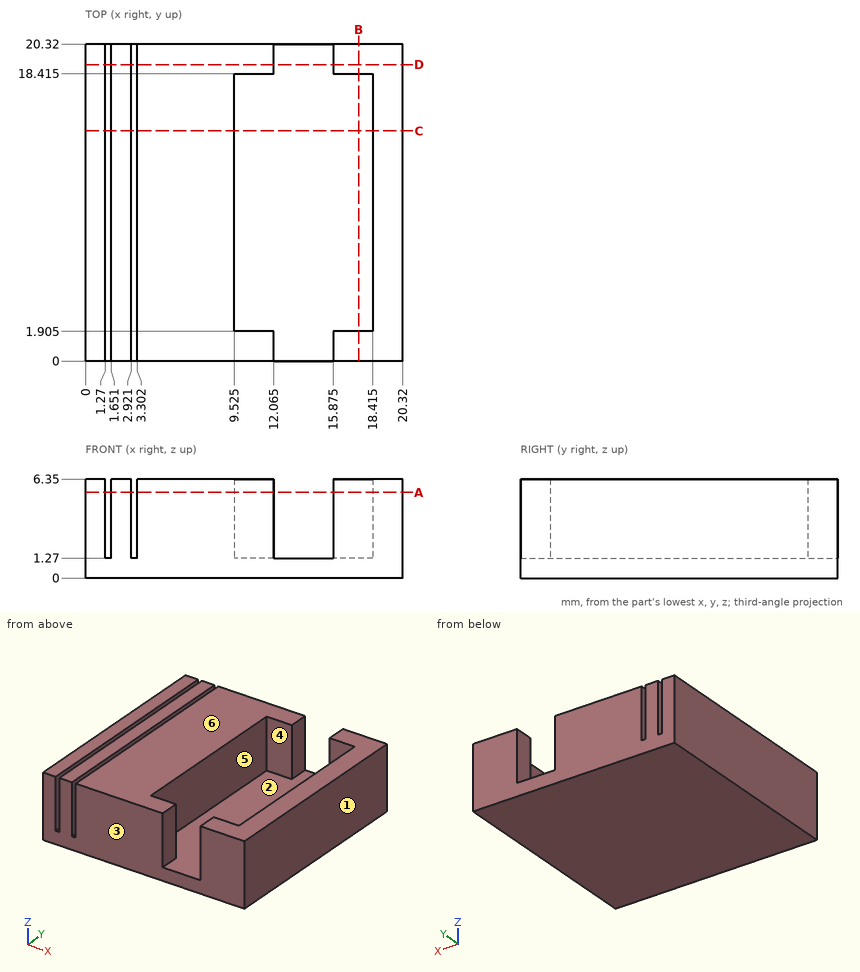
Check sheet for the drawn part. Datum: minimum x, y, z corner. Units: mm. A direction names the side the tool comes from. Give positions to 0.01 mm unless a question says otherwise; leave off trailing zeros. Order: outer loops, then holes, each group sorted by start corner. A loop starts at its lowest first (then second) coordinate and runs counter-clockwise, first axis right, second up. Notation, with made-up numbers: (66.5, -36) -> (83.5, -36) arc R17 ccw to (83.5, -18) -> close; hole circle Ø1 at (-38, -33). An arc over 180 degrees is marked (long way). Return JSON: item names as keys, results as strings.
1. Material ranges on probe 1 along X at (y, z) = (4.25, 5.5) (3 decimals); probe 2 along X at (y, z) = (19.75, 5.75) (3 decimals); probe 3 along Y at (x, z) = (10.5, 2) (3 decimals), recorded low to high. Write a range as [from, to].
From the geometry:
{"probe 1": "[0, 1.27], [1.651, 2.921], [3.302, 9.525], [18.415, 20.32]", "probe 2": "[0, 1.27], [1.651, 2.921], [3.302, 12.065], [15.875, 20.32]", "probe 3": "[0, 1.905], [18.415, 20.32]"}
2. Cross-section at D-D, the plane y = 19. Record the cut outline in (x, z) (3 decimals).
From the geometry:
{"outline": "(0, 0) -> (20.32, 0) -> (20.32, 6.35) -> (15.875, 6.35) -> (15.875, 1.27) -> (12.065, 1.27) -> (12.065, 6.35) -> (3.302, 6.35) -> (3.302, 1.27) -> (2.921, 1.27) -> (2.921, 6.35) -> (1.651, 6.35) -> (1.651, 1.27) -> (1.27, 1.27) -> (1.27, 6.35) -> (0, 6.35) -> close"}
3. Cross-section at A-A, the plane z = 5.5. Record the cut outline in (x, y) (3 decimals).
From the geometry:
{"outline": "(0, 0) -> (1.27, 0) -> (1.27, 20.32) -> (0, 20.32) -> close; (1.651, 0) -> (2.921, 0) -> (2.921, 20.32) -> (1.651, 20.32) -> close; (3.302, 0) -> (12.065, 0) -> (12.065, 1.905) -> (9.525, 1.905) -> (9.525, 18.415) -> (12.065, 18.415) -> (12.065, 20.32) -> (3.302, 20.32) -> close; (15.875, 0) -> (20.32, 0) -> (20.32, 20.32) -> (15.875, 20.32) -> (15.875, 18.415) -> (18.415, 18.415) -> (18.415, 1.905) -> (15.875, 1.905) -> close"}
4. Cross-section at B-B, the plane x = 17.5. Record the cut outline in (y, z) (3 decimals).
From the geometry:
{"outline": "(0, 0) -> (20.32, 0) -> (20.32, 6.35) -> (18.415, 6.35) -> (18.415, 1.27) -> (1.905, 1.27) -> (1.905, 6.35) -> (0, 6.35) -> close"}
5. Set-up check for the marked faces 5 and 6: record each of +Z, -Z, +X, -X, +Y, -Y from which the full face is reachable in a straight line by a thin tool's end or side.
From the geometry:
{"face 5": "+Z", "face 6": "+Z, +X, -X, +Y, -Y"}
6. Mould release check, pull along Y, two halves, no side actions. Record for the marked faces 1, 2, 3 and 4: +Y half, -Y half, draft (parallel to the pull), parting line (faces both ways), or undercut.
From the geometry:
{"face 1": "draft", "face 2": "undercut", "face 3": "-Y half", "face 4": "undercut"}
7. Go/stop test with a flat-tipped pin: P1, Ø5, axis at x = 14.5, y = 12, coming from the +Z side. Record where the tip stops, or that it passes through.
From the geometry:
{"P1": "z = 1.27"}
8. Cross-section at C-C, the plane y = 14.75. Record the cut outline in (x, z) (3 decimals).
From the geometry:
{"outline": "(0, 0) -> (20.32, 0) -> (20.32, 6.35) -> (18.415, 6.35) -> (18.415, 1.27) -> (9.525, 1.27) -> (9.525, 6.35) -> (3.302, 6.35) -> (3.302, 1.27) -> (2.921, 1.27) -> (2.921, 6.35) -> (1.651, 6.35) -> (1.651, 1.27) -> (1.27, 1.27) -> (1.27, 6.35) -> (0, 6.35) -> close"}
